Design review of the part built by this model. Coordinates are the model's own, in mm. A direction names the side the tool comes from. Give positions to 0.01 mm unless a question says otherwise; leave off trailing zeros. Write each loop counter-clockwise with the first axis right and the second up, starting at its lowest first coordinate (ties: lowest second). Pieces come first, ordered by that corner, then holes. Notation, with made-up numbers: (-26, 38.25) -> (-17, 38.25) arc R17 ccw to (-17, 61.25) -> close; hole circle Ø7 at (-4, 25). An arc over 180 degrees is marked (long way). Answer as a JSON object with one key per item and string values.
```python
from build123d import *

# Parameters (mm, degrees)
BOSS_EXTRUDE1_DEPTH   = 7
BOSS_EXTRUDE1_2_DEPTH = 7
BOSS_EXTRUDE2_DEPTH   = 15
CUT_EXTRUDE2_START    = 10
SKETCH3_R             = 92.486171345
SKETCH3_R_2           = 70
CUT_EXTRUDE2_DEPTH    = 10
CHAMFER2_SIZE         = 10
SKETCH4_R             = 4
CUT_EXTRUDE3_DEPTH    = 163.113620009
SKETCH5_R             = 11
CUT_EXTRUDE4_DEPTH    = 5
SKETCH6_R             = 2.5
CUT_EXTRUDE5_DEPTH    = 171.073513517
BOSS_EXTRUDE3_DEPTH   = 7


with BuildPart() as part:
    # Sketch1 → Boss-Extrude1 (new body)
    with BuildSketch(Plane(origin=(0, 0, 0), x_dir=(1, 0, 0), z_dir=(0, 1, 0))):
        with BuildLine():
            ThreePointArc((65.383484153, 25), (49.497474683, 49.497474683), (25, 65.383484153))
            Line((25, 65.383484153), (25, 25))
            Line((25, 25), (65.383484153, 25))
        make_face()
    extrude(amount=-BOSS_EXTRUDE1_DEPTH)



with BuildPart() as body_2:
    # Sketch1 → Boss-Extrude1 2 (new body)
    with BuildSketch(Plane(origin=(0, 0, 0), x_dir=(1, 0, 0), z_dir=(0, 1, 0))):
        with BuildLine():
            Line((25, -25), (25, -65.383484153))
            ThreePointArc((25, -65.383484153), (49.497474683, -49.497474683), (65.383484153, -25))
            Line((65.383484153, -25), (25, -25))
        make_face()
    extrude(amount=-BOSS_EXTRUDE1_2_DEPTH)


with BuildPart() as part_1:
    add(part.part)

    add(body_2.part)  # Boss-Extrude2 merges body 2
    # Sketch2 → Boss-Extrude2 (add)
    with BuildSketch(Plane.ZY.offset(-25)):
        with BuildLine():
            Line((-65.383484153, 0), (-93.894188194, 92.646921016))
            ThreePointArc((-93.894188194, 92.646921016), (-82.896855971, 121.416608183), (-52.324444318, 117.679783125))
            Line((-52.324444318, 117.679783125), (65.383484153, 0))
            Line((65.383484153, 0), (25, 0))
            Line((25, 0), (-42.366125313, 77.869487777))
            ThreePointArc((-42.366125313, 77.869487777), (-55.501453858, 79.630239272), (-58.849166194, 66.807216074))
            Line((-58.849166194, 66.807216074), (-25, 0))
            Line((-25, 0), (-65.383484153, 0))
        make_face()
    extrude(amount=-BOSS_EXTRUDE2_DEPTH)

    # Sketch3 → Cut-Extrude2 (cut)
    with BuildSketch(Plane(origin=(0, 0, 0), x_dir=(1, 0, 0), z_dir=(0, 1, 0)).offset(CUT_EXTRUDE2_START)):
        Circle(SKETCH3_R)
        Circle(SKETCH3_R_2, mode=Mode.SUBTRACT)
    extrude(amount=-CUT_EXTRUDE2_DEPTH, mode=Mode.SUBTRACT)

    # Chamfer2
    # the kernel refuses this chamfer: 10 mm, written as the material it adds along each edge
    with BuildSketch(Plane(origin=(0, 10, 0), x_dir=(0.8280566024533268, 0, -0.5606445069145448), z_dir=(0.5606445069145448, 0, 0.8280566024533268))) as chamfer2_piece_1_section:
        Polygon((70 + CHAMFER2_SIZE, 0), (70, -CHAMFER2_SIZE), (70, 0), align=None)
    chamfer2_piece_1 = revolve(axis=Axis((0, 10, 0), (0, 1, 0)), revolution_arc=56.024500162, mode=Mode.PRIVATE)
    chamfer2_piece_1 = split(chamfer2_piece_1, bisect_by=Plane(origin=(33.827146268, 0, -63.755868056), z_dir=(0, 1, 0)), keep=Keep.TOP, mode=Mode.PRIVATE)
    chamfer2_piece_1 = split(chamfer2_piece_1, bisect_by=Plane(origin=(40, 6.324094296, -63.755868056), z_dir=(-1, 0, 0)), keep=Keep.TOP, mode=Mode.PRIVATE)
    chamfer2_piece_1 = split(chamfer2_piece_1, bisect_by=Plane(origin=(33.827146268, 5.319462172, -67.020469063), z_dir=(0, 0.2941231593783912, 0.9557675277583318)), keep=Keep.TOP, mode=Mode.PRIVATE)
    chamfer2_piece_1 = split(chamfer2_piece_1, bisect_by=Plane(origin=(25, 6.324094296, -63.755868056), z_dir=(1, 0, 0)), keep=Keep.TOP, mode=Mode.PRIVATE)
    add(chamfer2_piece_1)

    # Sketch4 → Cut-Extrude3 (cut, through all)
    with BuildSketch(Plane.ZY.offset(-25)):
        with Locations((-70, 100)):
            Circle(SKETCH4_R)
    extrude(amount=-CUT_EXTRUDE3_DEPTH, mode=Mode.SUBTRACT)

    # Sketch5 → Cut-Extrude4 (cut)
    with BuildSketch(Plane.ZY.offset(-25)):
        with Locations((-70, 100)):
            Circle(SKETCH5_R)
    extrude(amount=-CUT_EXTRUDE4_DEPTH, mode=Mode.SUBTRACT)

    # Sketch6 → Cut-Extrude5 (cut, through all)
    with BuildSketch(Plane(origin=(0, 0, 0), x_dir=(1, 0, 0), z_dir=(0, 1, 0))):
        with Locations(Location((47.5, 35, 0), (0, 0, 270))):
            Circle(SKETCH6_R)
        with Locations(Location((47.5, -35, 0), (0, 0, 270))):
            Circle(SKETCH6_R)
    extrude(amount=-CUT_EXTRUDE5_DEPTH, mode=Mode.SUBTRACT)

    # Sketch7 → Boss-Extrude3 (add)
    with BuildSketch(Plane(origin=(0, 0, 0), x_dir=(1, 0, 0), z_dir=(0, 1, 0))):
        with BuildLine():
            Line((25, -65.383484153), (25.1277486, -48.924393203))
            ThreePointArc((25.1277486, -48.924393203), (20.356318028, -51.094229775), (15.4, -52.8))
            ThreePointArc((15.4, -52.8), (10.3, -62.1), (19.6, -67.2))
            ThreePointArc((19.6, -67.2), (22.318488579, -66.346703517), (25, -65.383484153))
        make_face()
    extrude(amount=-BOSS_EXTRUDE3_DEPTH)


solid = part_1.part
```
(1) We need section D-D, the plane z = 60. State the section outline as (x, y) points.
Here are the results:
{"outline": "(10, -7) -> (36.06, -7) -> (36.06, 5.38) -> (25, 5.38) -> (25, 0) -> (10, 0) -> close"}
(2) We need section B-B, the plane y = 61. State the section outline as (x, z) points, then the cut area to 3 significant figures.
Here are the results:
{"outline": "(25, -84.16) -> (40, -84.16) -> (40, -55.91) -> (25, -55.91) -> close; (25, -27.77) -> (40, -27.77) -> (40, 4.37) -> (25, 4.37) -> close", "area": "906 mm²"}
(3) For faces 1 (the flat face through (32.39, 38.39, -8.21)), 2 (the flat face through (17, 0, 60)), 3 (the flat face through (50, 0, 37)), 4 (the flat face through (45, -3, 25)), 5 (the flat face through (30, 95, -70)), list the 3-axis set-ups (+Z, -Z, +X, -X, +Y, -Y) from which the entire face can be reached by the end or side of a thin tool; tool diameter is ignored.
Here are the results:
{"face 1": "+X, -X", "face 2": "+Z, -Z, -X, +Y", "face 3": "+Z, -Z, +X, +Y", "face 4": "+X, -X, -Y", "face 5": "-X"}
(4) For line 1 along X through (y, z) = (77.5, -25.5); line 2 along Z through (x, y) = (27, 14.5); line 3 along Z through (x, y) = (37, 79), list the stretches that pass through material, from the lowest coordinate up.
Here are the results:
{"line 1": "x = 25 to 40", "line 2": "z = -69.85 to -32.35, 12.46 to 50.88", "line 3": "z = -89.69 to -56.34, -43.52 to -13.64"}
(5) The part is to be moulded in two halves that separate along Z. For faces 6 (the cylindrical face through (20.357, -3.451, 51.094)), 7 (the flat face through (32.39, 33.87, -42.16)), 8 (the flat face through (25, 45, -49)), say which applies: +Z half, -Z half, draft (parallel to the pull), parting line (faces both ways), or undercut.
Here are the results:
{"face 6": "-Z half", "face 7": "undercut", "face 8": "draft"}
(6) We need section C-C, the plane z = -35. State the section outline as (x, y) points.
Here are the results:
{"outline": "(25, -7) -> (45, -7) -> (45, 0) -> (40, 0) -> (40, 19.74) -> (25, 19.74) -> close; (25, 69.35) -> (40, 69.35) -> (40, 100.36) -> (25, 100.36) -> close; (50, -7) -> (60.62, -7) -> (60.62, 0) -> (50, 0) -> close"}
(7) Clearance check with flat-ended pins moving along their axes: pin 1 (24 mm diameter, centred on y = 104.5, z = -75, fed in from -X); pin 2 (5 mm diameter, centred on x = 25, y = 24.5, fed in from -Z); pin 3 (2 mm diameter, centred on x = 37, y = -2.5, fed in from -Z). State where each tip first meets the part, or that it passes through.
Here are the results:
{"pin 1": "stops at x = 25", "pin 2": "stops at z = -73.69", "pin 3": "stops at z = -60.03"}
(8) We need section A-A, the plane x = 57. State the section outline as (y, z) points.
Here are the results:
{"outline": "(-7, -40.63) -> (0, -40.63) -> (0, -25) -> (-7, -25) -> close; (-7, 25) -> (0, 25) -> (0, 40.63) -> (-7, 40.63) -> close"}
